```python
from build123d import *

# Parameters (mm, degrees)
SKETCH1_W           = 300
SKETCH1_H           = 304.8
BOSS_EXTRUDE1_DEPTH = 200
BOSS_EXTRUDE3_DEPTH = 304.8
SHELL1_T            = 3
CUT_EXTRUDE3_REACH  = 435.426
SKETCH8_R           = 2.65
CUT_EXTRUDE4_REACH  = 435.426
SKETCH9_R           = 1.5
SKETCH9_W           = 28
SKETCH9_H           = 19


with BuildPart() as part:
    # Sketch1 → Boss-Extrude1 (new body)
    with BuildSketch(Plane.XY):
        Rectangle(SKETCH1_W, SKETCH1_H)
    extrude(amount=-BOSS_EXTRUDE1_DEPTH)

    # Sketch7 → Boss-Extrude3 (add, through all)
    with BuildSketch(Plane.XZ.offset(152.4)):
        Polygon((-172, -200), (-172, -127.5), (-172, 0), (172, 0), (172, -127.5), (172, -200), align=None)
    extrude(amount=-BOSS_EXTRUDE3_DEPTH)

    # Sketch2 → Cut-Revolve1 (revolve, cut)
    with BuildSketch(Plane(origin=(0, 0, 0), x_dir=(1, 0, 0), z_dir=(0, 1, 0))):
        Polygon((0, 0), (135.5, 0), (135.5, 7), (118.5, 7), (111.799574733, 45), (0, 45), align=None)
    revolve(axis=Axis((0, 0, 0), (0, 0, -1)), mode=Mode.SUBTRACT)

    # Shell1
    shell1_openings = [part.faces().sort_by_distance(p)[0] for p in [
        (-115.149787367, 0, -26),
        (0, 0, -45),
    ]]
    offset(amount=SHELL1_T, openings=shell1_openings, kind=Kind.INTERSECTION)

    # Sketch8 → Cut-Extrude3 (cut, up to next)
    with BuildSketch(Plane.ZY.offset(175), mode=Mode.PRIVATE) as cut_extrude3_sk1:
        with Locations((-40.65, -121.75)):
            Circle(SKETCH8_R)
    cut_extrude3_tool1 = extrude(cut_extrude3_sk1.sketch, amount=-CUT_EXTRUDE3_REACH, mode=Mode.PRIVATE) & part.part
    # Sketch8 → Cut-Extrude3 (cut, up to next)
    with BuildSketch(Plane.ZY.offset(175), mode=Mode.PRIVATE) as cut_extrude3_sk2:
        with Locations((-22, -121.75)):
            Circle(SKETCH8_R)
    cut_extrude3_tool2 = extrude(cut_extrude3_sk2.sketch, amount=-CUT_EXTRUDE3_REACH, mode=Mode.PRIVATE) & part.part
    # Sketch8 → Cut-Extrude3 (cut, up to next)
    with BuildSketch(Plane.ZY.offset(175), mode=Mode.PRIVATE) as cut_extrude3_sk3:
        with Locations((-22, -140.4)):
            Circle(SKETCH8_R)
    cut_extrude3_tool3 = extrude(cut_extrude3_sk3.sketch, amount=-CUT_EXTRUDE3_REACH, mode=Mode.PRIVATE) & part.part
    # Sketch8 → Cut-Extrude3 (cut, up to next)
    with BuildSketch(Plane.ZY.offset(175), mode=Mode.PRIVATE) as cut_extrude3_sk4:
        with Locations((-40.65, -140.4)):
            Circle(SKETCH8_R)
    cut_extrude3_tool4 = extrude(cut_extrude3_sk4.sketch, amount=-CUT_EXTRUDE3_REACH, mode=Mode.PRIVATE) & part.part
    add(cut_extrude3_tool1.solids().sort_by_distance((-175, -121.75, -40.65))[0], mode=Mode.SUBTRACT)
    add(cut_extrude3_tool2.solids().sort_by_distance((-175, -121.75, -22))[0], mode=Mode.SUBTRACT)
    add(cut_extrude3_tool3.solids().sort_by_distance((-175, -140.4, -22))[0], mode=Mode.SUBTRACT)
    add(cut_extrude3_tool4.solids().sort_by_distance((-175, -140.4, -40.65))[0], mode=Mode.SUBTRACT)

    # Sketch9 → Cut-Extrude4 (cut, up to next)
    with BuildSketch(Plane(origin=(175, 0, 0), x_dir=(0, 0, -1), z_dir=(1, 0, 0)), mode=Mode.PRIVATE) as cut_extrude4_sk1:
        with Locations((8.68, -59.4)):
            Circle(SKETCH9_R)
    cut_extrude4_tool1 = extrude(cut_extrude4_sk1.sketch, amount=-CUT_EXTRUDE4_REACH, mode=Mode.PRIVATE) & part.part
    # Sketch9 → Cut-Extrude4 (cut, up to next)
    with BuildSketch(Plane(origin=(175, 0, 0), x_dir=(0, 0, -1), z_dir=(1, 0, 0)), mode=Mode.PRIVATE) as cut_extrude4_sk2:
        with Locations((49.32, -59.4)):
            Circle(SKETCH9_R)
    cut_extrude4_tool2 = extrude(cut_extrude4_sk2.sketch, amount=-CUT_EXTRUDE4_REACH, mode=Mode.PRIVATE) & part.part
    # Sketch9 → Cut-Extrude4 (cut, up to next)
    with BuildSketch(Plane(origin=(175, 0, 0), x_dir=(0, 0, -1), z_dir=(1, 0, 0)), mode=Mode.PRIVATE) as cut_extrude4_sk3:
        with Locations((29, -59.4)):
            Rectangle(SKETCH9_W, SKETCH9_H)
    cut_extrude4_tool3 = extrude(cut_extrude4_sk3.sketch, amount=-CUT_EXTRUDE4_REACH, mode=Mode.PRIVATE) & part.part
    add(cut_extrude4_tool1.solids().sort_by_distance((175, -59.4, -8.68))[0], mode=Mode.SUBTRACT)
    add(cut_extrude4_tool2.solids().sort_by_distance((175, -59.4, -49.32))[0], mode=Mode.SUBTRACT)
    add(cut_extrude4_tool3.solids().sort_by_distance((175, -59.4, -29))[0], mode=Mode.SUBTRACT)


solid = part.part
```
Verification items for the finished model (mm, model axes). A direction names the side the tool comes from. Coordinates: 2 decimals unless noted, no trailing zeros. Write each loop counter-clockwise with the first axis right and the second up, starting at its lowest first coordinate (ties: lowest second). Pieces come first, ordered by that corner, then holes. Notation, with made-up numbers: M 50.25,6.25 L 90.25,6.25 A11 ccw 90.25,15.25 Z; hole C 38.5,-8.5 d6. An arc over 180 degrees is marked long. Answer as a JSON object with one key per item and string values. Group by question number.
(1) Material ranges on line 1 (Y direction, x = -173.95, z = -22); line 2 (Z direction, x = -172.8, y = -140.4); line 3 (Y direction, x = 0, z = -1.75), recorded low to high.
(2) Release check for a two-part mould opening along Y. For faces 1 (the face through (2, 152.4, -99)), 2 (the face through (2, -2, -203)), 3 (the face through (2, 155.4, -99)) record: +Y half, -Y half, draft (parallel to the pull), parting line (faces both ways), or undercut.
(3) Cross-section at B-B, the plane x = 0. Record the cut outline in (y, z), and give its area (3 significant figures).
(4) Tool access check on faces 4 (the face through (-172, -2, -99)), 5 (the face through (-109, -50, -4)), 6 (the face through (2, -155.4, -99)). Record the directions out of +Z, -Z, +X, -X, +Y, -Y that give a thin tool (end or side, any length) a straight path to the whole face; none if there is none.
(5) Gauge pin test, flat ends, axial feed: pin 1 (1.8 mm diameter, centred on y = -59.4, z = -49.32, fed in from +X); pin 2 (3 mm diameter, centred on y = -140.4, z = -22, fed in from -X). Record the tip position at first contact, or that the pin passes through.
(6) Cross-section at A-A, the plane z = -138. Record the cut outline in (x, y).
(7) Cross-section at C-C, the plane x = -127.5. Record the cut outline in (y, z).
Reply:
{
 "1": {"line 1": "-155.4 to -143.05, -137.75 to -124.4, -119.1 to 155.4", "line 2": "-203 to -43.3, -38 to -24.65, -19.35 to 3", "line 3": "-155.4 to -152.4, -135.5 to -132.5, 132.5 to 135.5, 152.4 to 155.4"},
 "2": {"face 1": "undercut", "face 2": "draft", "face 3": "+Y half"},
 "3": {"outline": "M -155.4,-203 L 155.4,-203 L 155.4,3 L 132.5,3 L 132.5,-4 L 119.03,-4 L 118.5,-7 L 135.5,-7 L 135.5,0 L 152.4,0 L 152.4,-200 L -152.4,-200 L -152.4,0 L -135.5,0 L -135.5,-7 L -118.5,-7 L -119.03,-4 L -132.5,-4 L -132.5,3 L -155.4,3 Z", "area": "2,390 mm²"},
 "4": {"face 4": "none", "face 5": "+Z", "face 6": "+Z, -Z, +X, -X, -Y"},
 "5": {"pin 1": "x = -172", "pin 2": "x = 172"},
 "6": {"outline": "M -175,-155.4 L 175,-155.4 L 175,155.4 L -175,155.4 Z; hole M -172,-152.4 L 172,-152.4 L 172,152.4 L -172,152.4 Z"},
 "7": {"outline": "M -155.4,-203 L 155.4,-203 L 155.4,3 L 36.06,3 L 36.06,-4 L -36.06,-4 L -36.06,3 L -155.4,3 Z; hole M -152.4,-200 L 152.4,-200 L 152.4,0 L 45.87,0 L 45.87,-7 L -45.87,-7 L -45.87,0 L -152.4,0 Z"}
}
